```python
from build123d import *

# Parameters (mm, degrees)
POCKET_DEPTH = 1


with BuildPart() as part:
    # Sketch → Revolution (revolve)
    with BuildSketch(Plane.XY):
        with BuildLine():
            Line((0, -5.5), (1, -5.5))
            Line((1, -5.5), (1.4, -5.1))
            Line((1.4, -5.1), (1.4, 0))
            Line((1.4, 0), (1.961192, 0))
            ThreePointArc((1.961192, 0), (2.448253, 0.201747), (2.65, 0.688808))
            ThreePointArc((2.65, 0.688808), (2.265961, 1.615961), (1.338808, 2))
            Line((1.338808, 2), (0, 2))
            Line((0, 2), (0, -5.5))
        make_face()
    revolve(axis=Axis((0, 0, 0), (0, 1, 0)))

    # Sketch001 (on Face7 of Revolution) → Pocket (cut)
    with BuildSketch(Plane(origin=(0, 2, 0), x_dir=(-1, 0, 0), z_dir=(0, 1, 0))):
        Polygon((0.754634, 1.307064), (0, 1.158183), (-0.754634, 1.307064), (-1.003016, 0.579091), (-1.509267, 0), (-1.003016, -0.579091), (-0.754634, -1.307064), (0, -1.158183), (0.754634, -1.307064), (1.003016, -0.579091), (1.509267, 0), (1.003016, 0.579091), align=None)
    extrude(amount=-POCKET_DEPTH, mode=Mode.SUBTRACT)


solid = part.part
```
Input: part model. Units: mm. Frame: model coordinates. Give positions to 0.01 mm unless a question says otherwise; leave off trailing zeros. Order: outer loops, then holes, each group sorted by start corner. A loop starts at its lowest first (then second) coordinate and runs counter-clockwise, first axis right, second up.
1. Pin query (flat end, axial travel): pin 1 Ø2 at (y, z) = (1, 2) entering from +X; pin 2 Ø2 at (x, z) = (2, 2) entering from +Y; pin 3 Ø2 at (y, z) = (-1.5, 0) entering from +X. Return the tip coordinate at first contact, or that it passes through.
Computed:
pin 1: stops at x = 2.44
pin 2: stops at y = 1.91
pin 3: stops at x = 1.4
2. Draft query along X for faces 1 (the face through (0, 1, 0)), 2 (the face through (-1.3, 0, -0.9)), 3 (the face through (-1.4, -2.51, -0.06)). Return one class per face: released by +X, released by -X, zero draft, split by the parting line, or undercut.
Computed:
face 1: undercut
face 2: zero draft
face 3: split by the parting line
3. Line query: probe 1 along Z at (x, y) = (0, 0.75); probe 2 along Z at (x, y) = (0, -5); probe 3 along Y at (x, z) = (-0.4, -0.65). Output: solid intervals per line, ascending.
Computed:
probe 1: z = -2.65 to 2.65
probe 2: z = -1.4 to 1.4
probe 3: y = -5.5 to 1
4. Cut plane A-A (y = -4). Return loops of the section in (x, z), and give its area (3 significant figures).
Computed:
outline: circle Ø2.8 at (0, 0)
area: 6.16 mm2
